The listing builds one solid part. Answer for the finished solid, in the listing's coordinates (mm). A direction names the side the tool comes from. Round coordinates to 2 decimals unless told otherwise and drop trailing zeros. Order: outer loops, then holes, each group sorted by start corner. A loop starts at its lowest first (then second) coordinate and runs counter-clockwise, first axis right, second up. Notation, with made-up numbers: (56, -24.75) -> (112, -24.75) arc R20 ccw to (112, -11.75) -> close; hole circle Ø7 at (73.5, 74). An arc over 180 degrees is marked (long way). Answer in a Markdown table with one row per item. Add a question column.
```python
from build123d import *

# Parameters (mm, degrees)
EXTRUDE_1_DEPTH     = 50
SKETCH_3_R          = 6
CUT_EXTRUDE_1_DEPTH = 50
SKETCH_4_R          = 1.8
CUT_EXTRUDE_2_DEPTH = 28
CHAMFER_1_SIZE      = 1.5
CUT_EXTRUDE_3_DEPTH = 12
CUT_EXTRUDE_START   = -5
CUT_EXTRUDE_4_DEPTH = 9
SKETCH_10_R         = 3.25
CUT_EXTRUDE_5_DEPTH = 80
CHAMFER_2_SIZE      = 6
SKETCH_11_R         = 2.2
EXTRUDE_2_DEPTH     = 8
EXTRUDE_3_DEPTH     = 8
EXTRUDE_4_DEPTH     = 4
EXTRUDE_6_DEPTH     = 8
CHAMFER_3_SIZE      = 10
CHAMFER_4_SIZE      = 12
CHAMFER_5_SIZE      = 2
FILLET_1_R          = 8
SKETCH_17_R         = 4.05
CUT_EXTRUDE_6_DEPTH = 3
FILLET_2_R          = 0.5


with BuildPart() as part:
    # 草图1 → 凸台-拉伸1 (new body)
    with BuildSketch(Plane.XY):
        Polygon((33, 0), (-33, 0), (-33, 80), (-25, 80), (-25, 4), (25, 4), (25, 80), (33, 80), align=None)
    extrude(amount=EXTRUDE_1_DEPTH)

    # 草图3 → 切除-拉伸1 (cut)
    with BuildSketch(Plane.XZ):
        with Locations(Location((0, 25, 0), (0, 0, 270))):
            Circle(SKETCH_3_R)
    extrude(amount=-CUT_EXTRUDE_1_DEPTH, mode=Mode.SUBTRACT)

    # 草图4 → 切除-拉伸2 (cut)
    with BuildSketch(Plane.XZ):
        with Locations(Location((0, 40, 0), (0, 0, 270))):
            Circle(SKETCH_4_R)
        with Locations(Location((15, 25, 0), (0, 0, 270))):
            Circle(SKETCH_4_R)
        with Locations(Location((0, 10, 0), (0, 0, 270))):
            Circle(SKETCH_4_R)
        with Locations(Location((-15, 25, 0), (0, 0, 270))):
            Circle(SKETCH_4_R)
    extrude(amount=-CUT_EXTRUDE_2_DEPTH, mode=Mode.SUBTRACT)

    # 倒角1
    chamfer_1_edges = [part.edges().sort_by_distance(p)[0] for p in [
        (0, 4, 41.8),
        (15, 4, 26.8),
        (0, 4, 11.8),
        (-15, 4, 26.8),
    ]]
    chamfer(chamfer_1_edges, length=CHAMFER_1_SIZE)

    # 草图6 → 切除-拉伸3 (cut)
    with BuildSketch(Plane.ZY.offset(33)):
        with BuildLine():
            Line((13.8, 20), (13.8, 23))
            ThreePointArc((13.8, 23), (25, 34.2), (36.2, 23))
            Line((36.2, 23), (36.2, 20))
            ThreePointArc((36.2, 20), (25, 8.8), (13.8, 20))
        make_face()
        with BuildLine():
            Line((11.15, 38), (11.15, 36))
            ThreePointArc((11.15, 36), (9.5, 34.35), (7.85, 36))
            Line((7.85, 36), (7.85, 38))
            ThreePointArc((7.85, 38), (9.5, 39.65), (11.15, 38))
        make_face()
        with BuildLine():
            Line((38.85, 38), (38.85, 36))
            ThreePointArc((38.85, 36), (40.5, 34.35), (42.15, 36))
            Line((42.15, 36), (42.15, 38))
            ThreePointArc((42.15, 38), (40.5, 39.65), (38.85, 38))
        make_face()
        with BuildLine():
            Line((11.15, 5), (11.15, 7))
            ThreePointArc((11.15, 7), (9.5, 8.65), (7.85, 7))
            Line((7.85, 7), (7.85, 5))
            ThreePointArc((7.85, 5), (9.5, 3.35), (11.15, 5))
        make_face()
        with BuildLine():
            Line((38.85, 5), (38.85, 7))
            ThreePointArc((38.85, 7), (40.5, 8.65), (42.15, 7))
            Line((42.15, 7), (42.15, 5))
            ThreePointArc((42.15, 5), (40.5, 3.35), (38.85, 5))
        make_face()
    cut_extrude_3 = extrude(amount=-CUT_EXTRUDE_3_DEPTH, mode=Mode.SUBTRACT)

    # 草图9 → 切除-拉伸4 (cut)
    with BuildSketch(Plane.ZY.offset(33).offset(CUT_EXTRUDE_START)):
        with BuildLine():
            Line((12.4, 38), (12.4, 36))
            ThreePointArc((12.4, 36), (9.5, 33.1), (6.6, 36))
            Line((6.6, 36), (6.6, 38))
            ThreePointArc((6.6, 38), (9.5, 40.9), (12.4, 38))
        make_face()
        with BuildLine():
            Line((37.6, 38), (37.6, 36))
            ThreePointArc((37.6, 36), (40.5, 33.1), (43.4, 36))
            Line((43.4, 36), (43.4, 38))
            ThreePointArc((43.4, 38), (40.5, 40.9), (37.6, 38))
        make_face()
        with BuildLine():
            Line((37.6, 5), (37.6, 7))
            ThreePointArc((37.6, 7), (40.5, 9.9), (43.4, 7))
            Line((43.4, 7), (43.4, 5))
            ThreePointArc((43.4, 5), (40.5, 2.1), (37.6, 5))
        make_face()
        with BuildLine():
            Line((12.4, 5), (12.4, 7))
            ThreePointArc((12.4, 7), (9.5, 9.9), (6.6, 7))
            Line((6.6, 7), (6.6, 5))
            ThreePointArc((6.6, 5), (9.5, 2.1), (12.4, 5))
        make_face()
    cut_extrude_4 = extrude(amount=-CUT_EXTRUDE_4_DEPTH, mode=Mode.SUBTRACT)

    # 镜向1: 切除-拉伸3, 切除-拉伸4 across plane
    add(cut_extrude_3.mirror(Plane(origin=(0, 0, 0), x_dir=(0, 0, 1), z_dir=(1, 0, 0))), mode=Mode.SUBTRACT)
    add(cut_extrude_4.mirror(Plane(origin=(0, 0, 0), x_dir=(0, 0, 1), z_dir=(1, 0, 0))), mode=Mode.SUBTRACT)

    # 草图10 → 切除-拉伸5 (cut)
    with BuildSketch(Plane(origin=(33, 0, 0), x_dir=(0, 0, -1), z_dir=(1, 0, 0))):
        with Locations(Location((-25, 68.5, 0), (0, 0, 90))):
            Circle(SKETCH_10_R)
    extrude(amount=-CUT_EXTRUDE_5_DEPTH, mode=Mode.SUBTRACT)

    # 倒角2
    chamfer_2_edges = [part.edges().sort_by_distance(p)[0] for p in [
        (29, 80, 50),
    ]]
    chamfer(chamfer_2_edges, length=CHAMFER_2_SIZE)

    # 草图11 → 凸台-拉伸2 (add)
    with BuildSketch(Plane(origin=(33, 0, 0), x_dir=(0, 0, -1), z_dir=(1, 0, 0))):
        Polygon((-50, 63.445571485), (-50, 74), (-44, 80), (-44, 92), (-62, 92), (-62, 74), (-62, 54.790404535), (-50, 54.790404535), align=None)
        with Locations(Location((-55.310889132, 86, 0), (0, 0, 90))):
            Circle(SKETCH_11_R, mode=Mode.SUBTRACT)
    extrude(amount=-EXTRUDE_2_DEPTH)

    # 草图13 → 凸台-拉伸3 (add)
    with BuildSketch(Plane.ZY.offset(33)):
        Polygon((50, 80), (80, 30), (80, 0), (50, 0), align=None)
    extrude_3 = extrude(amount=-EXTRUDE_3_DEPTH)

    # 镜向2: 凸台-拉伸3 across plane
    add(extrude_3.mirror(Plane(origin=(0, 0, 0), x_dir=(0, 0, 1), z_dir=(1, 0, 0))))

    # 草图14 → 凸台-拉伸4 (add)
    with BuildSketch(Plane.XZ):
        Polygon((-25, 80), (-15, 50), (-25, 50), align=None)
    extrude_4 = extrude(amount=-EXTRUDE_4_DEPTH)

    # 镜向3: 凸台-拉伸4 across plane
    add(extrude_4.mirror(Plane(origin=(0, 0, 0), x_dir=(0, 0, 1), z_dir=(1, 0, 0))))

    # 草图16 → 凸台-拉伸6 (add)
    with BuildSketch(Plane.ZY.offset(33)):
        Polygon((0, 25), (-11, 7), (-11, 0), (0, 0), align=None)
    extrude_6 = extrude(amount=-EXTRUDE_6_DEPTH)

    # 镜向5: 凸台-拉伸6 across plane
    add(extrude_6.mirror(Plane(origin=(0, 0, 0), x_dir=(0, 0, 1), z_dir=(1, 0, 0))))

    # 倒角3
    chamfer_3_edges = [part.edges().sort_by_distance(p)[0] for p in [
        (29, 80, 0),
        (-29, 80, 0),
    ]]
    chamfer(chamfer_3_edges, length=CHAMFER_3_SIZE)

    # 倒角4
    chamfer_4_edges = [part.edges().sort_by_distance(p)[0] for p in [
        (29, 80, 44),
    ]]
    chamfer(chamfer_4_edges, length=CHAMFER_4_SIZE - 0.0001)  # a hair under: the kernel refuses the full size

    # 倒角5
    chamfer_5_edges = [part.edges().sort_by_distance(p)[0] for p in [
        (29, 92, 62),
    ]]
    chamfer(chamfer_5_edges, length=CHAMFER_5_SIZE)

    # 圆角1
    fillet_1_edges = [part.edges().sort_by_distance(p)[0] for p in [
        (-29, 80, 50),
    ]]
    fillet(fillet_1_edges, radius=FILLET_1_R)

    # 草图17 → 切除-拉伸6 (cut)
    with BuildSketch(Plane.ZY.offset(-25)):
        with Locations(Location((55.310889132, 86, 0), (0, 0, 270))):
            Circle(SKETCH_17_R)
    extrude(amount=-CUT_EXTRUDE_6_DEPTH, mode=Mode.SUBTRACT)

    # 圆角2
    fillet_2_edges = [part.edges().sort_by_distance(p)[0] for p in [
        (25, 90.05, 55.310889132),
    ]]
    fillet(fillet_2_edges, radius=FILLET_2_R)


solid = part.part
```
Item 1: The part is cut by section A-A, the plane y = 68.5. Give the vertices of the cut face in (x, z), and give its area (3 significant figures).
Item 2: The part is cut by section C-C, the plane y = 44. Give the vertices of the cut face in (x, z), and give its area (3 significant figures).
Item 3: The part is cut by section B-B, the plane x = 0. Give the vertices of the cut face in (y, z).
Item 4: Flat-ended cylindrical pins translate along their axes: P1, Ø0.6, axis at x = 29.5, y = 37, coming from the -Z side; P2, Ø4, axis at y = 68.5, z = 25, coming from the -X side; P3, Ø6, axis at x = 22.5, y = 75.5, coming from the -Z side; P4, Ø2, axis at x = 30.5, y = 37.5, coming from the +Z side. Find the tip coordinate at first contact, or state that the pin passes through.
Item 5: For a pull along Y with two mould halves and no side action, classify faces 1 (the face through (-30.54, 8.65, 40.46)), 2 (the face through (-29, 15, 80)), 3 (the face through (29, 86, 38)) as released by +Y, released by -Y, zero draft, split by the parting line, or undercut.
Item 6: The part is cut by section D-D, the plane z = 15. Give the vertices of the cut face in (x, y), and give its area (3 significant figures).
Item 7: A tool of negligible diameter and unlimited length cuts with its end or side. For faces 4 (the face through (-30.54, 39.65, 40.54)), 5 (the face through (28, 37.1, 7.6)), 6 (the face through (20, 2, 65)), 7 (the face through (30.54, 3.35, 9.46)), from which of +Z, -Z, +X, -X, +Y, -Y can it reach the whole face along a straight path? Write none if from no direction.
Item 8: Find the intervals of material crossed by probe 1 along Z at (x, y) = (27.4, 86); probe 2 along Z at (x, y) = (27.5, 68.5); probe 3 along X at (y, z) = (39.5, 65.5), in increasing order. Write a range as [from, to].
Resolved:
| question | item | result |
|---|---|---|
| 1 | outline | (-33, 0) -> (-25, 0) -> (-25, 21.75) -> (-33, 21.75) -> close; (-33, 28.25) -> (-25, 28.25) -> (-25, 56.9) -> (-33, 56.9) -> close; (25, 0) -> (33, 0) -> (33, 21.75) -> (25, 21.75) -> close; (25, 28.25) -> (33, 28.25) -> (33, 62) -> (25, 62) -> close |
| 1 | area | 847 mm2 |
| 2 | outline | (-33, 0) -> (-25, 0) -> (-25, 71.6) -> (-33, 71.6) -> close; (25, 0) -> (33, 0) -> (33, 71.6) -> (25, 71.6) -> close |
| 2 | area | 1,150 mm2 |
| 3 | outline | (0, 0) -> (4, 0) -> (4, 6.7) -> (2.5, 8.2) -> (0, 8.2) -> close; (0, 11.8) -> (2.5, 11.8) -> (4, 13.3) -> (4, 19) -> (0, 19) -> close; (0, 31) -> (4, 31) -> (4, 36.7) -> (2.5, 38.2) -> (0, 38.2) -> close; (0, 41.8) -> (2.5, 41.8) -> (4, 43.3) -> (4, 50) -> (0, 50) -> close |
| 4 | P1 | z = 0 |
| 4 | P2 | through |
| 4 | P3 | z = 3.84 |
| 4 | P4 | z = 76.1 |
| 5 | face 1 | undercut |
| 5 | face 2 | zero draft |
| 5 | face 3 | released by +Y |
| 6 | outline | (-33, 0) -> (33, 0) -> (33, 14.96) -> (25, 14.96) -> (25, 4) -> (-25, 4) -> (-25, 14.96) -> (-33, 14.96) -> close; (-33, 28.04) -> (-25, 28.04) -> (-25, 80) -> (-33, 80) -> close; (25, 28.04) -> (33, 28.04) -> (33, 80) -> (25, 80) -> close |
| 6 | area | 1,270 mm2 |
| 7 | face 4 | +X, -X |
| 7 | face 5 | none |
| 7 | face 6 | +Z, +Y, -Y |
| 7 | face 7 | +X |
| 8 | probe 1 | [38, 51.26], [59.36, 62] |
| 8 | probe 2 | [0, 21.75], [28.25, 62] |
| 8 | probe 3 | [-33, -25], [25, 33] |
